The listing builds one solid part. Answer for the finished solid, in the listing's coordinates (mm). Face numbers are marked on the shaded views. A direction names the side the tool comes from. Coordinates: 2 decimals unless noted, no trailing zeros. Order: outer loops, then holes, each group sorted by start corner. A loop starts at its lowest first (then second) coordinate and runs counter-clockwise, first axis right, second up. Notation, with made-up numbers: (23.5, -33.75) -> (60.5, -33.75) arc R14 cw to (60.5, -16.75) -> close; hole circle Ø5 at (31, 55). An arc over 180 degrees is marked (long way). Answer in a Markdown table with one row per item. Add a question column.
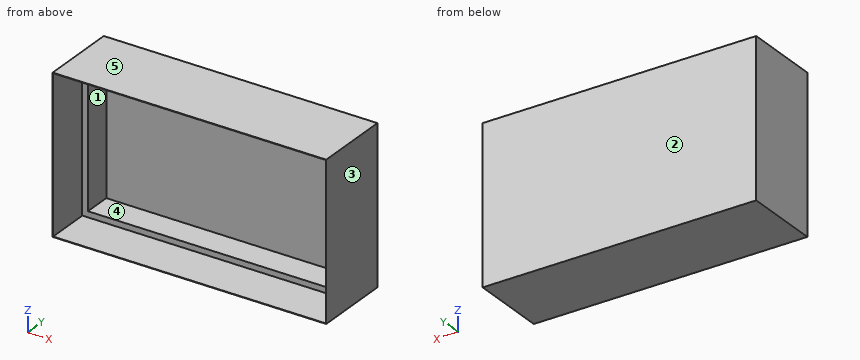
```python
from build123d import *

# Parameters (mm, degrees)
F0_W     = 118.8842207193
F0_H     = 67.5890743732
F1_DEPTH = 33.3094447851
F2_T     = -0.2
F3_W     = 118.2425096631
F3_H     = 66.9943261892
F4_DEPTH = 14.4755076617
F5_T     = -2.54


with BuildPart() as f1:
    # F0 (on Front) → F1 (new body)
    with BuildSketch(Plane.XZ):
        Rectangle(F0_W, F0_H)
    extrude(amount=F1_DEPTH)

    # F2
    f2_openings = [f1.faces().sort_by_distance(p)[0] for p in [
        (0, -33.309445, 0),
    ]]
    offset(amount=F2_T, openings=f2_openings)

    # F3 (on Front) → F4 (join)
    with BuildSketch(Plane.XZ):
        with Locations((-0.072285533, 0.0539822504)):
            Rectangle(F3_W, F3_H)
    extrude(amount=F4_DEPTH)

    # F5
    f5_openings = [f1.faces().sort_by_distance(p)[0] for p in [
        (0, -16.754722, 33.594537),
        (-0.072286, -14.475508, 0.053982),
    ]]
    offset(amount=F5_T, openings=f5_openings)


solid = f1.part
```
Q1. A cutting plane is placed at C-C (y = -18). Determine the outline of the cut face in (x, z), then the cut area to 3 significant figures.
Q2. For the marked faces 1 and 2, determine the directions among +Z, -Z, +X, -X, +Y, -Y from which every point of the face is accessible in a straight line to the end or side of a thin tool.
Q3. Determine the mould class of the marked faces 3, 4 and 5 for opening direction X: +X half, -X half, draft (parallel to the pull), parting line (faces both ways), or undercut.
Q4. A cutting plane is placed at D-D (x = 3.5). Determine the outline of the cut face in (y, z), then the cut area to 3 significant figures.
Q5. A cutting plane is placed at A-A (y = -6.5). Determine the outline of the cut face in (x, z), then the cut area to 3 significant figures.
Q6. Given pin 1 (20 mm diameter, centred on x = -20, z = -4, fed in from -Y); pin 2 (10 mm diameter, centred on x = -24, z = -17.5, fed in from +Y), each flat-ended and moving along its own axis, determine where each tip first touches the part or whether it passes through.
Q7. Straight lines are drawn through the part: line 1 (X direction, y = -20, z = 9.5); line 2 (Z direction, x = 24, y = -30); line 3 (Y direction, x = 27, z = 18). For each, find the intervals that lie inside material, in ascending order.
Q8. A cutting plane is placed at B-B (z = -6.5). Determine the outline of the cut face in (x, y), then the cut area to 3 significant figures.
Returned:
| question | item | result |
|---|---|---|
| 1 | outline | (-59.44, -33.79) -> (59.44, -33.79) -> (59.44, 33.79) -> (-59.44, 33.79) -> close; hole (-59.24, -33.59) -> (59.24, -33.59) -> (59.24, 33.59) -> (-59.24, 33.59) -> close |
| 1 | area | 74.4 mm² |
| 2 | face 1 | -Y |
| 2 | face 2 | +Z, -Z, +X, -X, +Y |
| 3 | face 3 | +X half |
| 3 | face 4 | undercut |
| 3 | face 5 | draft |
| 4 | outline | (-33.31, -33.79) -> (0, -33.79) -> (0, 33.79) -> (-33.31, 33.79) -> (-33.31, 33.59) -> (-0.2, 33.59) -> (-0.2, 33.55) -> (-14.48, 33.55) -> (-14.48, 31.01) -> (-2.54, 31.01) -> (-2.54, -30.9) -> (-14.48, -30.9) -> (-14.48, -33.44) -> (-0.2, -33.44) -> (-0.2, -33.59) -> (-33.31, -33.59) -> close |
| 4 | area | 244 mm² |
| 5 | outline | (-59.44, -33.79) -> (59.44, -33.79) -> (59.44, 33.79) -> (-59.44, 33.79) -> close; (-59.19, -33.44) -> (59.05, -33.44) -> (59.05, 33.55) -> (-59.19, 33.55) -> close; hole (-59.24, -33.59) -> (59.24, -33.59) -> (59.24, 33.59) -> (-59.24, 33.59) -> close; hole (-56.65, -30.9) -> (56.51, -30.9) -> (56.51, 31.01) -> (-56.65, 31.01) -> close |
| 5 | area | 990 mm² |
| 6 | pin 1 | stops at y = -2.54 |
| 6 | pin 2 | stops at y = 0 |
| 7 | line 1 | x = -59.44 to -59.24, 59.24 to 59.44 |
| 7 | line 2 | z = -33.79 to -33.59, 33.59 to 33.79 |
| 7 | line 3 | y = -2.54 to 0 |
| 8 | outline | (-59.44, -33.31) -> (-59.24, -33.31) -> (-59.24, -0.2) -> (-59.19, -0.2) -> (-59.19, -14.48) -> (-56.65, -14.48) -> (-56.65, -2.54) -> (56.51, -2.54) -> (56.51, -14.48) -> (59.05, -14.48) -> (59.05, -0.2) -> (59.24, -0.2) -> (59.24, -33.31) -> (59.44, -33.31) -> (59.44, 0) -> (-59.44, 0) -> close |
| 8 | area | 374 mm² |
